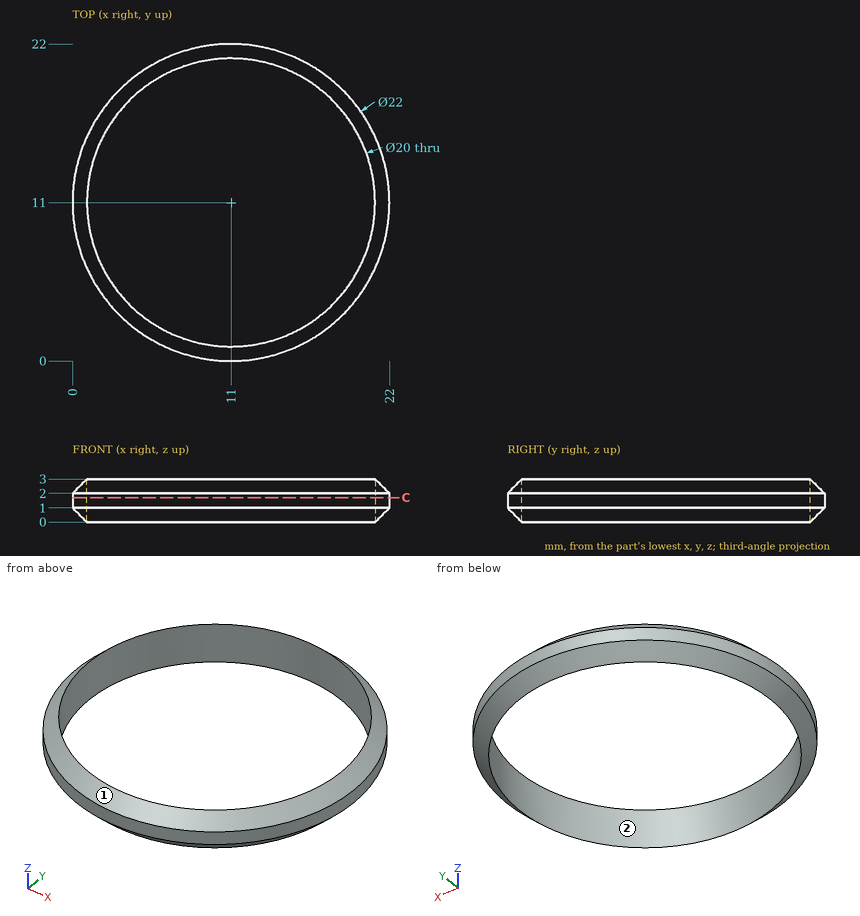
Print and shaded views of the part. All mm, measured from the part's lowest x, y and z. Round coordinates to 2 decimals unless told otherwise and drop trailing zeros. Loops run counter-clockwise (first coordinate to the right, second up) from the corner with the lowest first, then second, coordinate; pieces in that order, holes last. Notation, with made-up numbers: M 2,-0.5 L 19,-0.5 A19 cw 19,20.5 Z; hole C 43,82.25 d11. An arc over 180 degrees is marked long. One line per question, with ' | ' between items.
1) Drill centre lines: line 1 along Y through (x, z) = (19, 0.85); line 2 along Y through (x, z) = (12, 0.35); line 3 along X through (y, z) = (6.25, 1.55). Where is each one in solid material? Low to high.
Solved:
line 1: y = 3.67 to 5, 17 to 18.33 | line 2: y = 0.7 to 1.05, 20.95 to 21.3 | line 3: x = 1.08 to 2.2, 19.8 to 20.92
2) Flat gauge pins, fed straight in: pin 1 (1.5 mm diameter, centred on x = 7.5, z = 0.5, fed in from -Y); pin 2 (1 mm diameter, centred on x = 3.5, y = 5, fed in from +Z). Where does each tip first touch, or does it go through?
Solved:
pin 1: stops at y = 0.4 | pin 2: stops at z = 3
3) Mould opens along Y. For the marked faces 1 and 2 say: +Y half, -Y half, draft (parallel to the pull), parting line (faces both ways), or undercut.
Solved:
face 1: parting line | face 2: undercut
4) Band-saw the part on C-C (z = 1.7). Give the cut face in (x, y), then the cut area to 3 significant figures.
Solved:
outline: C 11,11 d22; hole C 11,11 d20 | area: 66.0 mm²
